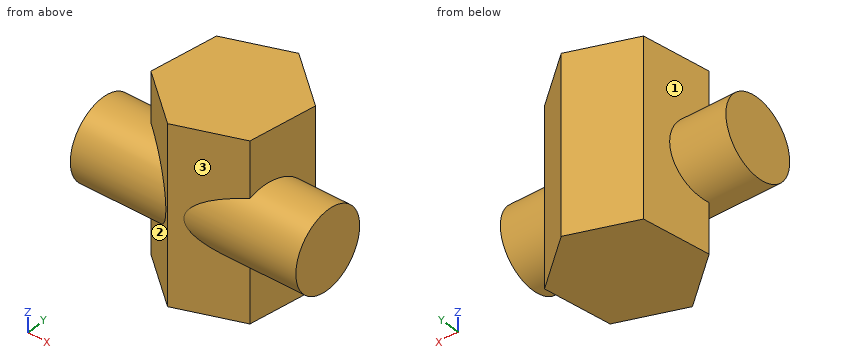
```python
from build123d import *

# Parameters (mm, degrees)
F1_DEPTH = 40
F2_R     = 17.5
F3_DEPTH = 50


with BuildPart() as f1:
    # F0 (on Top) → F1 (new body, symmetric)
    with BuildSketch(Plane.XY):
        Polygon((28.1907786236, 10.2606042998), (5.20944533, 29.5442325904), (-22.9813332936, 19.2836282906), (-28.1907786236, -10.2606042998), (-5.20944533, -29.5442325904), (22.9813332936, -19.2836282906), align=None)
    extrude(amount=F1_DEPTH, both=True)

    # F2 (on Right) → F3 (join, symmetric)
    with BuildSketch(Plane.YZ):
        with Locations((-10, 0)):
            Circle(F2_R)
    extrude(amount=F3_DEPTH, both=True)


solid = f1.part
```
Design review of the part built by this model. Coordinates are the model's own, in mm. Face numbers are marked on the shaded views. A direction names the side the tool comes from. Round coordinates to 2 decimals unless told otherwise and drop trailing zeros. Write each loop counter-clockwise with the first axis right and the second up, starting at its lowest first coordinate (ties: lowest second). Pieces come first, ordered by that corner, then holes. Notation, with made-up numbers: (-27, 87.25) -> (1, 87.25) arc R30 cw to (1, 118.25) -> close; hole circle Ø8 at (-20.5, -31.5). An arc over 180 degrees is marked (long way). Write item = value, one per line. Start each with the question number.
1) Wall thickness on probe 1 along X at (y, z) = (10.5, -18); probe 2 along Y at (x, z) = (-14, -26); probe 3 along Z at (x, y) = (-27.5, -11.5): over which ranges is each line inside the solid? List them lowest first. Write a range as from..to.
2) Take a section at A-A, the plane z = 21. State the section outline as (x, y) points.
3) Take a section at D-D, the plane z = 2. State the section outline as (x, y) points.
4) Tool access review of the marked faces 1, 2 and 3: name each direction out of +Z, -Z, +X, -X, +Y, -Y from which nothing blocks a thin tool from reaching the whole face with its end or side.
5) Clearance check with flat-ended pins moving along their axes: pin 1 (8 mm diameter, centred on x = 14.5, z = 2.5, fed in from +Y); pin 2 (10 mm diameter, centred on y = 21.5, z = 16, fed in from +X); pin 3 (1.5 mm diameter, centred on x = -39.5, y = 4.5, fed in from +Z). State where each tip first meets the part, or that it passes through.
6) Take a section at B-B, the plane y = -17. State the section outline as (x, z) points.
7) Take a section at C-C, the plane x = 30. State the section outline as (y, z) points.
Results list:
q1.probe_1 = -24.53..27.91
q1.probe_2 = -22.17..22.55
q1.probe_3 = -17.44..17.44
q2.outline = (-28.19, -10.26) -> (-5.21, -29.54) -> (22.98, -19.28) -> (28.19, 10.26) -> (5.21, 29.54) -> (-22.98, 19.28) -> close
q3.outline = (-50, -27.39) -> (-7.78, -27.39) -> (-5.21, -29.54) -> (0.72, -27.39) -> (50, -27.39) -> (50, 7.39) -> (27.68, 7.39) -> (28.19, 10.26) -> (5.21, 29.54) -> (-22.98, 19.28) -> (-25.08, 7.39) -> (-50, 7.39) -> close
q4.face_1 = -X, +Y
q4.face_2 = -X, -Y
q4.face_3 = +X, -Y
q5.pin_1 = 25.1
q5.pin_2 = 20.75
q5.pin_3 = 10.83
q6.outline = (-50, -16.04) -> (-20.16, -16.04) -> (-20.16, -40) -> (23.38, -40) -> (23.38, -16.04) -> (50, -16.04) -> (50, 16.04) -> (23.38, 16.04) -> (23.38, 40) -> (-20.16, 40) -> (-20.16, 16.04) -> (-50, 16.04) -> close
q7.outline = circle Ø35 at (-10, 0)
